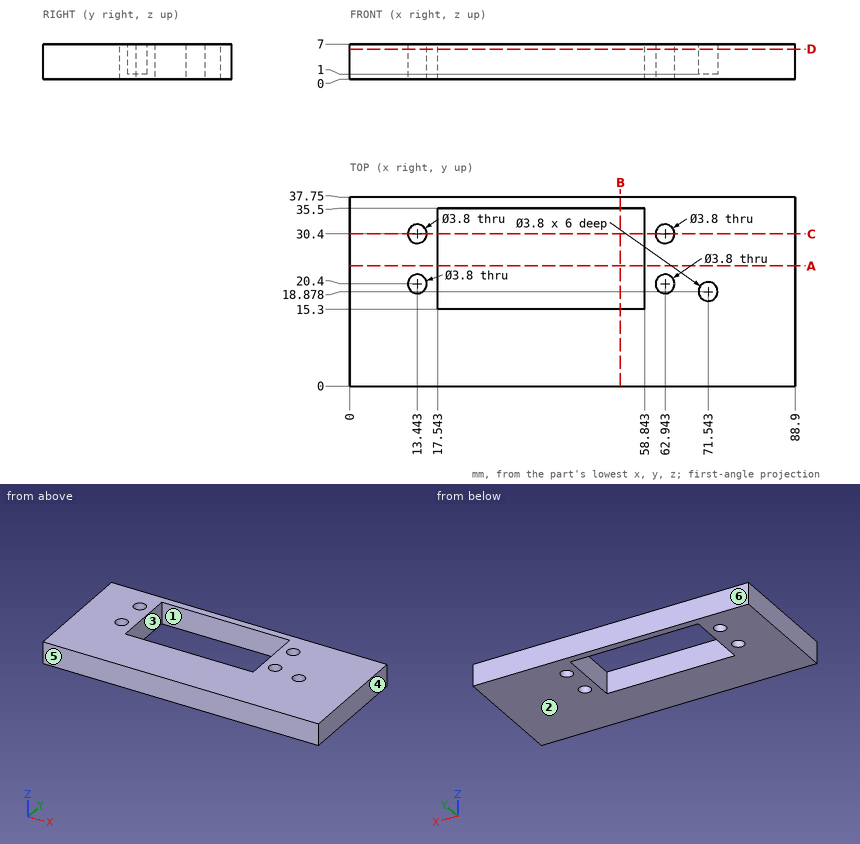
Job drawing, mm, ordinate dimensions from the low corner. One solid piece. A direction names the side the tool comes from. Round coordinates to 2 decimals unless told otherwise and drop trailing zeros. Write each loop counter-clockwise with the first axis right and the second up, starting at its lowest first coordinate (ties: lowest second). Pieces come first, ordered by that corner, then holes. Notation, with made-up numbers: (24.5, 13.5) -> (56.5, 13.5) arc R32 cw to (56.5, 40.5) -> close; hole circle Ø9 at (62.5, -14.5). An arc over 180 degrees is marked (long way). Answer as a JSON object with one key per item and string values.
(1) Two-plate mould, pull along Y, no slides. Class the marked faces 3, 4, 5 and 6: +Y half, -Y half, draft (parallel to the pull), parting line (faces both ways), or undercut.
Reported:
{"face 3": "undercut", "face 4": "draft", "face 5": "-Y half", "face 6": "+Y half"}
(2) Band-saw the part on D-D, the plane z = 6. List the corners of the cut face in (x, y), then the cut area to 4 significant figures.
Reported:
{"outline": "(0, 0) -> (88.9, 0) -> (88.9, 37.75) -> (0, 37.75) -> close; hole circle Ø3.8 at (13.44, 20.4); hole circle Ø3.8 at (13.44, 30.4); hole (17.54, 15.3) -> (58.84, 15.3) -> (58.84, 35.5) -> (17.54, 35.5) -> close; hole circle Ø3.8 at (62.94, 20.4); hole circle Ø3.8 at (62.94, 30.4); hole circle Ø3.8 at (71.54, 18.88)", "area": "2,465 mm^2"}
(3) Which spindle directions (+Z, -Z, +X, -X, +Y, -Y) get a long thin tool onto all of the face, cutting with end or side? Do the marked faces 1 and 2. Say none if no direction does.
Reported:
{"face 1": "+Z, -Z", "face 2": "-Z, +X, -X, +Y, -Y"}
(4) Probe probe 1 along Y at (x, z) = (23, 4); probe 2 along X at (y, z) = (33, 0.75); probe 3 along Y at (x, z) = (14.5, 0.75). List the from-to ranges inside material, lowest first. Write a range as [from, to].
Reported:
{"probe 1": "y = [0, 15.3], [35.5, 37.75]", "probe 2": "x = [0, 17.54], [58.84, 88.9]", "probe 3": "y = [0, 18.82], [21.98, 28.82], [31.98, 37.75]"}
(5) Band-saw the part on A-A, the plane y = 24. List the corners of the cut face in (x, z).
Reported:
{"outline": "(0, 0) -> (17.54, 0) -> (17.54, 7) -> (0, 7) -> close; (58.84, 0) -> (88.9, 0) -> (88.9, 7) -> (58.84, 7) -> close"}
(6) Band-saw the part on B-B, the plane x = 54. List the corners of the cut face in (y, z).
Reported:
{"outline": "(0, 0) -> (15.3, 0) -> (15.3, 7) -> (0, 7) -> close; (35.5, 0) -> (37.75, 0) -> (37.75, 7) -> (35.5, 7) -> close"}
(7) Band-saw the part on C-C, the plane y = 30.4. List the corners of the cut face in (x, z), then the cut area to 3 significant figures.
Reported:
{"outline": "(0, 0) -> (11.54, 0) -> (11.54, 7) -> (0, 7) -> close; (15.34, 0) -> (17.54, 0) -> (17.54, 7) -> (15.34, 7) -> close; (58.84, 0) -> (61.04, 0) -> (61.04, 7) -> (58.84, 7) -> close; (64.84, 0) -> (88.9, 0) -> (88.9, 7) -> (64.84, 7) -> close", "area": "280 mm^2"}
